Check sheet for the drawn part. Datum: minimum x, y, z corner. Units: mm. A direction names the side the tool comes from. Coordinates: 2 decimals unless noted, no trailing zeros. Loops run counter-clockwise (first coordinate to the right, second up) from the corner with the lowest first, then second, coordinate; pieces in that order, holes last.
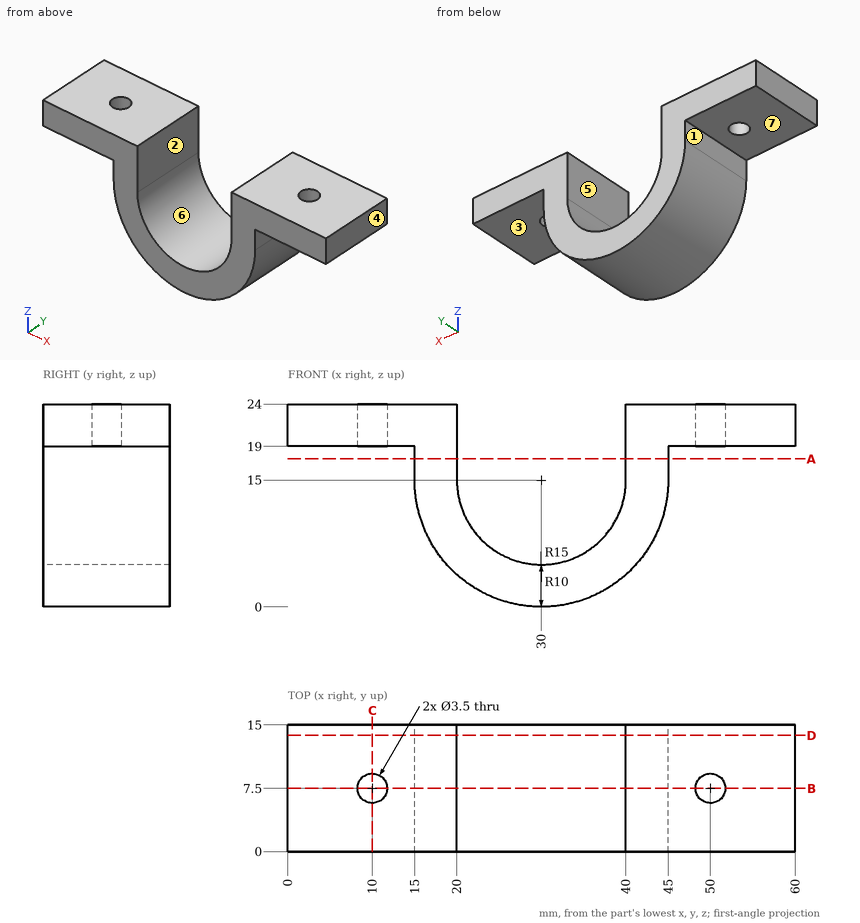
1) Section check B-B on y = 7.5. Enter the section's corners in (x, z), plus the area to 3 significant figures.
Answer sheet:
outline: (0, 19) - (8.25, 19) - (8.25, 24) - (0, 24) - close; (11.75, 19) - (15, 19) - (15, 15) arc R15 ccw to (45, 15) - (45, 19) - (48.25, 19) - (48.25, 24) - (40, 24) - (40, 15) arc R10 cw to (20, 15) - (20, 24) - (11.75, 24) - close; (51.75, 19) - (60, 19) - (60, 24) - (51.75, 24) - close
area: 401 mm2
2) Mould release check, pull along X, two halves, no side actions. Record for the marked faces 4, 5, 6 and 7: +X half, -X half, draft (parallel to the pull), parting line (faces both ways), or undercut.
Answer sheet:
face 4: +X half
face 5: undercut
face 6: undercut
face 7: draft
3) Depth check by flat-ended pin: pin 1 (1 mm diameter, centred on y = 3, z = 16, fed in from +X); pin 2 (4 mm diameter, centred on x = 53, z = 20, fed in from -Y); pin 3 (4 mm diameter, centred on x = 47.5, y = 5.5, fed in from -Z); pin 4 (4.5 mm diameter, centred on y = 8.5, z = 16, fed in from -X). Enter the tip coordinate at first touch or a pass-through.
Answer sheet:
pin 1: stops at x = 45
pin 2: stops at y = 0
pin 3: stops at z = 19
pin 4: stops at x = 15
4) Set-up check for the marked faces 1, 2 and 3: record each of +Z, -Z, +X, -X, +Y, -Y from which the full face is reachable in a straight line by a thin tool's end or side.
Answer sheet:
face 1: -Z, -X, +Y, -Y
face 2: +Z, +Y, -Y
face 3: -Z, +X, +Y, -Y
5) Scan lines: line 1 (X direction, y = 4.75, z = 17.75); line 2 (Y direction, x = 50, z = 21.9); line 3 (Z direction, x = 30, y = 3). Record each from-to range of solid material in increasing order.
Answer sheet:
line 1: x = 15 to 20, 40 to 45
line 2: y = 0 to 5.75, 9.25 to 15
line 3: z = 0 to 5
6) Section check A-A on z = 17.5. Enter the section's corners in (x, y).
Answer sheet:
outline: (15, 0) - (20, 0) - (20, 15) - (15, 15) - close; (40, 0) - (45, 0) - (45, 15) - (40, 15) - close
7) Section check D-D on y = 13.75. Enter the section's corners in (x, z).
Answer sheet:
outline: (0, 19) - (15, 19) - (15, 15) arc R15 ccw to (45, 15) - (45, 19) - (60, 19) - (60, 24) - (40, 24) - (40, 15) arc R10 cw to (20, 15) - (20, 24) - (0, 24) - close
8) Section check C-C on x = 10. Enter the section's corners in (y, z), plus the area to 3 significant figures.
Answer sheet:
outline: (0, 19) - (5.75, 19) - (5.75, 24) - (0, 24) - close; (9.25, 19) - (15, 19) - (15, 24) - (9.25, 24) - close
area: 57.5 mm2
